Part model, mm, in its own coordinate system. Face numbers are marked on the shaded views. A direction names the side the tool comes from. Give positions to 0.01 mm unless a question says otherwise; leave off trailing zeros. Write each loop counter-clockwise with the first axis right and the second up, starting at its lowest first coordinate (ties: lowest second). Pieces come first, ordered by that corner, then holes.
```python
from build123d import *

# Parameters (mm, degrees)
F1_DEPTH       = 0.5
F2_R           = 2.5
F3_DEPTH       = 0.3
F4_R           = 2.695
F5_DEPTH       = 3.2
F7_D           = 3
F7_DEPTH       = 3
F7_CSINK_D     = 4
F7_CSINK_ANGLE = 90
F7_TIP         = 0.9012909285


with BuildPart() as f1:
    # F0 (on Top) → F1 (new body)
    with BuildSketch(Plane.XY):
        Polygon((-2.7712812921, -1.6), (0, -3.2), (2.7712812921, -1.6), (2.7712812921, 1.6), (0, 3.2), (-2.7712812921, 1.6), align=None)
    extrude(amount=F1_DEPTH)

    # F2 (on face) → F3 (join)
    with BuildSketch(Plane.XY.offset(0.5)):
        Circle(F2_R)
    extrude(amount=F3_DEPTH)

    # F4 (on face) → F5 (join)
    with BuildSketch(Plane.XY.offset(0.8)):
        Circle(F4_R)
    extrude(amount=F5_DEPTH)

    # F7
    with Locations(Plane.XY.offset(4)):
        with Locations((0, 0)):
            CounterSinkHole(F7_D / 2, F7_CSINK_D / 2, depth=F7_DEPTH, counter_sink_angle=F7_CSINK_ANGLE)
            with Locations((0, 0, -(F7_DEPTH + F7_TIP / 2))):  # 118° drill point
                Cone(0, F7_D / 2, F7_TIP, mode=Mode.SUBTRACT)


solid = f1.part
```
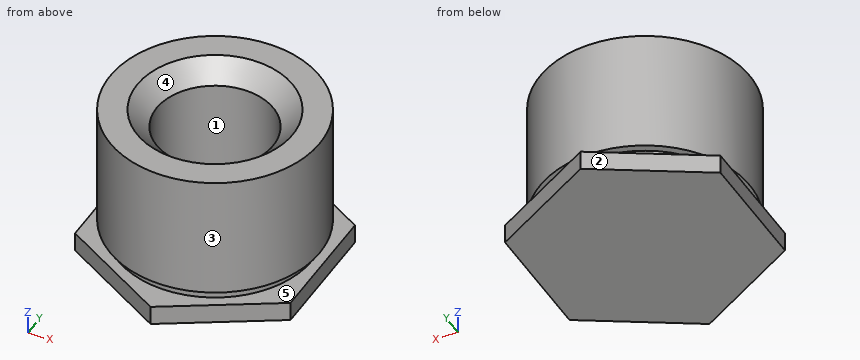
1) Wall check: L1, parallel to Y at x = 0, z = 2 (3 decimals); L2, parallel to Z at x = -0.9, y = 2.5; L3, parallel to Y at x = -1.3, z = 1.45. Give the ranges that are in metal, low to high.
Answers follow:
L1: y = -2.695 to -1.5, 1.5 to 2.695
L2: z = 0 to 0.5, 0.8 to 4
L3: y = -2.36 to -0.75, 0.75 to 2.36
2) Two-plate mould, pull along Y, no slides. Class the marked faces 3, 4 and 5: +Y half, -Y half, draft (parallel to the pull), parting line (faces both ways), or undercut.
Answers follow:
face 3: parting line
face 4: undercut
face 5: draft
3) Saw through at B-B, the plane x = 2.3. Write the cut outline in (y, z), then the cut area to 3 significant figures.
Answers follow:
outline: (-1.87, 0) - (1.87, 0) - (1.87, 0.5) - (0.98, 0.5) - (0.98, 0.8) - (1.4, 0.8) - (1.4, 4) - (-1.4, 4) - (-1.4, 0.8) - (-0.98, 0.8) - (-0.98, 0.5) - (-1.87, 0.5) - close
area: 11.4 mm2
4) Pin check, flat tips, straight feed: pin 1 Ø1 at (y, z) = (0, 1.5) entering from +X (3 decimals); pin 2 Ø2 at (x, y) = (2, -1) entering from -Z. Stop position of each tip, or through.
Answers follow:
pin 1: stops at x = 2.695
pin 2: stops at z = 0
5) 3-axis set-ups, long thin cutter, end or side, ignore diameter. For the marked faces 1 and 2: which of +Z, -Z, +X, -X, +Y, -Y reach the whole face in a straight line?
Answers follow:
face 1: +Z
face 2: +Z, -Z, -X, +Y
6) Saw through at A-A, the plane z = 3.4. Write the cut outline in (x, y) (3 decimals).
Answers follow:
outline: circle Ø5.39 at (0, 0); hole circle Ø3 at (0, 0)
